```python
from build123d import *

# Parameters (mm, degrees)
EXTRUDE_1_DEPTH     = 20
SKETCH_2_W          = 10
SKETCH_2_H          = 35
CUT_EXTRUDE_1_DEPTH = 112.915146428
EXTRUDE_START       = -35
SKETCH_3_W          = 40
SKETCH_3_H          = 15
EXTRUDE_2_DEPTH     = 70
SKETCH_4_R          = 6
CUT_EXTRUDE_2_DEPTH = 110.772492001
EXTRUDE_3_DEPTH     = 10


with BuildPart() as part:
    # Эскиз1 → Бобышка-Вытянуть1 (new body)
    with BuildSketch(Plane(origin=(0, 0, 0), x_dir=(0, 0, -1), z_dir=(1, 0, 0))):
        with BuildLine():
            Line((-35, 50), (-35, -50))
            Line((-35, -50), (-12.5, -50))
            Line((-12.5, -50), (-12.5, -38))
            Line((-12.5, -38), (12.5, -38))
            Line((12.5, -38), (12.5, -50))
            Line((12.5, -50), (35, -50))
            Line((35, -50), (35, 50))
            ThreePointArc((35, 50), (0, 15), (-35, 50))
        make_face()
        with BuildLine():
            ThreePointArc((35, 50), (0, 85), (-35, 50))
            Line((-35, 50), (-7.5, 50))
            ThreePointArc((-7.5, 50), (0, 57.5), (7.5, 50))
            Line((7.5, 50), (35, 50))
        make_face()
        with BuildLine():
            Line((-7.5, 50), (-35, 50))
            ThreePointArc((-35, 50), (0, 15), (35, 50))
            Line((35, 50), (7.5, 50))
            ThreePointArc((7.5, 50), (0, 42.5), (-7.5, 50))
        make_face()
    extrude(amount=-EXTRUDE_1_DEPTH)

    # Эскиз2 → Вырез-Вытянуть1 (cut, through all)
    with BuildSketch(Plane(origin=(0, 0, -35), x_dir=(-1, 0, 0), z_dir=(0, 0, -1))):
        with Locations((5, -2.5)):
            Rectangle(SKETCH_2_W, SKETCH_2_H)
    extrude(amount=-CUT_EXTRUDE_1_DEPTH, mode=Mode.SUBTRACT)

    # Эскиз3 → Бобышка-Вытянуть2 (add)
    with BuildSketch(Plane.XY.offset(EXTRUDE_START)):
        with Locations((-40, 7.5)):
            Rectangle(SKETCH_3_W, SKETCH_3_H)
    extrude(amount=EXTRUDE_2_DEPTH)

    # Эскиз4 → Вырез-Вытянуть2 (cut, through all)
    with BuildSketch(Plane.XZ):
        with Locations((-40, 0)):
            Circle(SKETCH_4_R)
    extrude(amount=-CUT_EXTRUDE_2_DEPTH, mode=Mode.SUBTRACT)

    # Эскиз5 → Бобышка-Вытянуть3 (add)
    with BuildSketch(Plane.XY.offset(35)):
        Polygon((-60, 15), (-20, 50), (-20, 15), align=None)
    extrude_3 = extrude(amount=-EXTRUDE_3_DEPTH)

    # Зеркальное отражение1: Бобышка-Вытянуть3 across plane
    add(extrude_3.mirror(Plane.XY))


solid = part.part
```
Can you work these out from the model? Positions are in its coordinate system, mm. A direction names the side the tool comes from. Give positions to 0.01 mm unless a question says otherwise; leave off trailing zeros. Order: outer loops, then holes, each group sorted by start corner. A loop starts at its lowest first (then second) coordinate and runs counter-clockwise, first axis right, second up. Notation, with made-up numbers: M 87.5,82.25 L 126.5,82.25 A28 cw 126.5,106.25 Z; hole C -18,47.25 d2. An arc over 180 degrees is marked long. Write item = value, one per line. Start each with the question number.
Q1. Will these pins go through, and if not, where does the flat tip stop? pin 1 Ø4 at (x, z) = (-10.5, -3) entering from -Y; pin 2 Ø1 at (y, z) = (-29.5, -8.5) entering from +X; pin 3 Ø8 at (x, z) = (-4.5, -2) entering from +Y; pin 4 Ø1.5 at (x, z) = (-21, 10.5) entering from -Y.
Q2. For faces 1 (the flat face through (-31, 25, -25)), 2 (the flat face through (-5, -20, 0)), 3 (the flat face through (-10, -44, -12.5)), 4 (the cylindrical face through (-9.86, 57.32, 1.63)), which set-ups out of +Z, -Z, +X, -X, +Y, -Y let a thin tool reach every point of the face, with its end or its side?
Q3. Suppose I cut it at A-A (x = -40). Write out the boundary of the cut face in (y, z).
Q4. Suppose I cut it at B-B (z = 0). Write out the boundary of the cut face in (x, y), plus the area to 3 significant figures.
Q5. I need wall thicknesses on probe 1 along Y at (x, z) = (-5, 0); probe 2 along Z at (x, y) = (-23.5, 30.5); probe 3 along Y at (x, z) = (-11, 0). Which ranges of each line are inside material? Lowest first, please. Write a range as [from, to].
Q6. We'd pull the mould along Z, two halves only. Please class faces 5 (the flat face through (-40, 0, -8)), 6 (the flat face through (-10, -44, 12.5)), 7 (the cylindrical face through (-9.86, 84.99, -0.77)): pulls with the +Z half, pulls with the -Z half, needs draft (parallel to the pull), parting line crosses it, or undercut.
Q7. Suppose I cut it at C-C (y = 44). Write out the boundary of the cut face in (x, z), plus the area to 3 significant figures.
Q8. Suppose I cut it at D-D (z = 21). Write out the boundary of the cut face in (x, y).
Check result:
q1.pin_1 = -38
q1.pin_2 = 0
q1.pin_3 = 85
q1.pin_4 = 0
q2.face_1 = -X, +Y
q2.face_2 = +Z, -Z, +X
q2.face_3 = +X, -X, -Y
q2.face_4 = +X, -X
q3.outline = M 0,-35 L 32.5,-35 L 32.5,-25 L 15,-25 L 15,-6 L 0,-6 Z; M 0,6 L 15,6 L 15,25 L 32.5,25 L 32.5,35 L 0,35 Z
q4.outline = M -60,0 L -46,0 L -46,15 L -60,15 Z; M -34,0 L -20,0 L -20,-38 L 0,-38 L 0,-20 L -10,-20 L -10,15 L 0,15 L 0,42.5 L -20,42.5 L -20,15 L -34,15 Z; M -20,57.5 L 0,57.5 L 0,85 L -20,85 Z
q4.area = 2,230 mm2
q5.probe_1 = [-38, -20], [15, 42.5], [57.5, 85]
q5.probe_2 = [-35, -25], [25, 35]
q5.probe_3 = [-38, 42.5], [57.5, 85]
q6.face_5 = needs draft
q6.face_6 = undercut
q6.face_7 = parting line crosses it
q7.outline = M -26.86,-35 L 0,-35 L 0,-4.5 L -20,-4.5 L -20,-25 L -26.86,-25 Z; M -26.86,25 L -20,25 L -20,4.5 L 0,4.5 L 0,35 L -26.86,35 Z
q7.area = 1,360 mm2
q8.outline = M -60,0 L -20,0 L -20,-50 L 0,-50 L 0,-20 L -10,-20 L -10,15 L 0,15 L 0,78 L -20,78 L -20,15 L -60,15 Z
